The model under review builds one solid part; all positions refer to its coordinate system, in mm. Face numbers are marked on the shaded views. A direction names the side the tool comes from. Give positions to 0.01 mm unless a question says otherwise; leave off trailing zeros. Loops run counter-clockwise (first coordinate to the right, second up) from the corner with the lowest first, then second, coordinate; pieces in that order, holes last. Notation, with made-up numbers: M 15.25,-6.5 L 44.25,-6.5 A12 ccw 44.25,11.5 Z; hole C 41.5,54 d5. An arc over 180 degrees is marked long. Return JSON: item names as keys, results as strings.
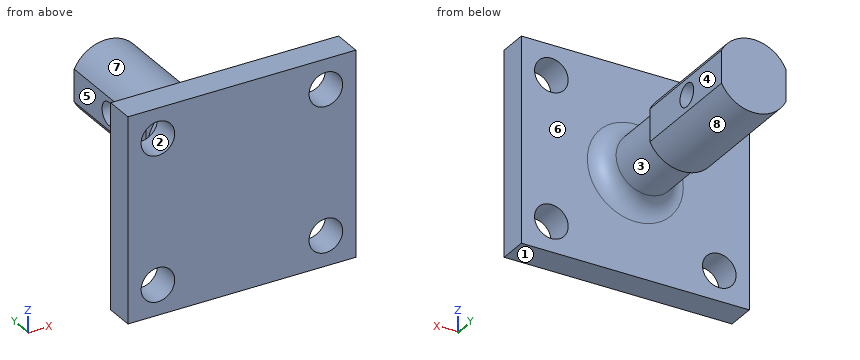
```python
from build123d import *

# Parameters (mm, degrees)
SKETCH1_W               = 9.5
SKETCH1_H               = 8.5
BOSS_EXTRUDE1_DEPTH     = 1.2
CUT_EXTRUDE1_DEPTH      = 7.485753619
CUT_EXTRUDE1_DEPTH_BACK = 7.485753619
SKETCH2_R               = 0.7
SKETCH5_R               = 1.25
BOSS_EXTRUDE2_DEPTH     = 3.25
FILLET1_R               = 0.75
SKETCH37_R              = 1.5
BOSS_EXTRUDE3_DEPTH     = 5
CUT_EXTRUDE3_START      = -6
CUT_EXTRUDE3_DEPTH      = 6
SKETCH41_R              = 0.475
CUT_EXTRUDE4_DEPTH      = 10


with BuildPart() as part:
    # Sketch1 → Boss-Extrude1 (new body)
    with BuildSketch(Plane(origin=(0, 0, 0), x_dir=(1, 0, 0), z_dir=(0, 1, 0))):
        Rectangle(SKETCH1_W, SKETCH1_H)
    extrude(amount=BOSS_EXTRUDE1_DEPTH)

    # Sketch2 → Cut-Extrude1 (cut, two sides: drawn at the far end of the back side and taken through both)
    with BuildSketch(Plane(origin=(0, 1.2, 0), x_dir=(1, 0, 0), z_dir=(0, 1, 0)).offset(-CUT_EXTRUDE1_DEPTH_BACK)):
        with Locations(Location((-3.5, -3, 0), (0, 0, 270))):
            Circle(SKETCH2_R)
        with Locations(Location((-3.5, 3, 0), (0, 0, 270))):
            Circle(SKETCH2_R)
        with Locations(Location((3.5, 3, 0), (0, 0, 270))):
            Circle(SKETCH2_R)
        with Locations(Location((3.5, -3, 0), (0, 0, 270))):
            Circle(SKETCH2_R)
    extrude(amount=CUT_EXTRUDE1_DEPTH + CUT_EXTRUDE1_DEPTH_BACK, mode=Mode.SUBTRACT)

    # Sketch5 → Boss-Extrude2 (add)
    with BuildSketch(Plane(origin=(0, 1.2, 0), x_dir=(1, 0, 0), z_dir=(0, 1, 0))):
        with Locations(Location((0, 0, 0), (0, 0, 90))):
            Circle(SKETCH5_R)
    extrude(amount=BOSS_EXTRUDE2_DEPTH)

    # Fillet1
    fillet1_edges = [part.edges().sort_by_distance(p)[0] for p in [
        (0, 1.2, 1.25),
    ]]
    fillet(fillet1_edges, radius=FILLET1_R)

    # Sketch37 → Boss-Extrude3 (add)
    with BuildSketch(Plane(origin=(0, 4.45, 0), x_dir=(1, 0, 0), z_dir=(0, 1, 0))):
        with Locations(Location((0, 0, 0), (0, 0, 270))):
            Circle(SKETCH37_R)
    extrude(amount=BOSS_EXTRUDE3_DEPTH)

    # Sketch40 → Cut-Extrude3 (cut)
    with BuildSketch(Plane(origin=(0, 9.45, 0), x_dir=(1, 0, 0), z_dir=(0, 1, 0)).offset(CUT_EXTRUDE3_START)):
        with BuildLine():
            Line((-1.339542832, 0.675), (-1.339542832, -0.675))
            ThreePointArc((-1.339542832, -0.675), (-1.5, 0), (-1.339542832, 0.675))
        make_face()
        with BuildLine():
            Line((1.339542832, 0.675), (1.339542832, -0.675))
            ThreePointArc((1.339542832, -0.675), (1.5, 0), (1.339542832, 0.675))
        make_face()
    extrude(amount=CUT_EXTRUDE3_DEPTH, mode=Mode.SUBTRACT)

    # Sketch41 → Cut-Extrude4 (cut)
    with BuildSketch(Plane(origin=(1.339542832, 0, 0), x_dir=(0, 0, -1), z_dir=(1, 0, 0))):
        with Locations((0, 7.03)):
            Circle(SKETCH41_R)
    extrude(amount=-CUT_EXTRUDE4_DEPTH, mode=Mode.SUBTRACT)


solid = part.part
```
1) The part is to be moulded in two halves that separate along X. For the marked faces 1, 2 and 3, say which applies: released by +X, released by -X, zero draft, split by the parting line, or undercut.
From the geometry:
{"face 1": "zero draft", "face 2": "undercut", "face 3": "split by the parting line"}
2) Tool access review of the marked faces 4, 5, 6, 7 and 8: name each direction out of +Z, -Z, +X, -X, +Y, -Y from which nothing blocks a thin tool from reaching the whole face with its end or side.
From the geometry:
{"face 4": "+Z, -Z, +X, +Y", "face 5": "+Z, -Z, -X, +Y", "face 6": "+Y", "face 7": "+Z, +Y", "face 8": "-Z, +Y"}
3) Wall thickness on L1, parallel to X at y = 1, z = -3; L2, parallel to Z at x = 3.5, y = 0.9; L3, parallel to Y at x = 0.65, z = 0 (3 decimals): over which ranges is each line inside the solid? List them lowest first. Write a range as from..to.
From the geometry:
{"L1": "-4.75..-4.2, -2.8..2.8, 4.2..4.75", "L2": "-4.25..-3.7, -2.3..2.3, 3.7..4.25", "L3": "0..6.555, 7.505..9.45"}
4) Consider section D-D on x = 0. Write out the cut boundary in (y, z) (3 decimals), then the cut area to 3 significant figures.
From the geometry:
{"outline": "M 0,-4.25 L 1.2,-4.25 L 1.2,-2 A0.75 cw 1.95,-1.25 L 4.45,-1.25 L 4.45,-1.5 L 9.45,-1.5 L 9.45,1.5 L 4.45,1.5 L 4.45,1.25 L 1.95,1.25 A0.75 cw 1.2,2 L 1.2,4.25 L 0,4.25 Z; hole C 7.03,0 d0.95", "area": "32.9 mm²"}
5) Insertion check: pin 1 (5 mm diameter, centred on x = -3, y = 6.5, fed in from -Z); pin 2 (1.5 mm diameter, centred on x = -2, y = 6.5, fed in from -Z); pin 3 (0.7 mm diameter, centred on y = 7, z = 0.5, fed in from -X). Each pin has a flat end and moves straight along its axis. Give the tip position at first contact, or say it passes through.
From the geometry:
{"pin 1": "z = -1.41", "pin 2": "z = -0.83", "pin 3": "x = -1.34"}
6) Consider section A-A on z = 3. Write out the cut boundary in (x, y).
From the geometry:
{"outline": "M -4.75,0 L -4.2,0 L -4.2,1.2 L -4.75,1.2 Z; M -2.8,0 L 2.8,0 L 2.8,1.2 L -2.8,1.2 Z; M 4.2,0 L 4.75,0 L 4.75,1.2 L 4.2,1.2 Z"}
7) Consider section B-B on x = 3.5. Write out the cut boundary in (y, z), then the cut area to 3 significant figures.
From the geometry:
{"outline": "M 0,-4.25 L 1.2,-4.25 L 1.2,-3.7 L 0,-3.7 Z; M 0,-2.3 L 1.2,-2.3 L 1.2,2.3 L 0,2.3 Z; M 0,3.7 L 1.2,3.7 L 1.2,4.25 L 0,4.25 Z", "area": "6.84 mm²"}
8) Consider section C-C on z = 0. Write out the cut boundary in (x, y) (3 decimals), then the cut area to 3 significant figures.
From the geometry:
{"outline": "M -4.75,0 L 4.75,0 L 4.75,1.2 L 2,1.2 A0.75 cw 1.25,1.95 L 1.25,4.45 L 1.34,4.45 L 1.34,6.555 L -1.34,6.555 L -1.34,4.45 L -1.25,4.45 L -1.25,1.95 A0.75 cw -2,1.2 L -4.75,1.2 Z; M -1.34,7.505 L 1.34,7.505 L 1.34,9.45 L -1.34,9.45 Z", "area": "30.6 mm²"}
